Verification items for the finished model (mm, model axes). Coordinates: 2 decimals unless noted, no trailing zeros. Loops run counter-clockwise (first coordinate to the right, second up) from the corner with the lowest first, then second, coordinate; pieces in that order, holes last. Notation, with made-up numbers: (-16, 46.5) - (6, 46.5) arc R14 ccw to (6, 69.5) - close; hole circle Ø10 at (67.25, -30). An arc over 180 degrees is marked (long way). Answer as CSV lines item,"result". Start each with the question number.
1. Release check for a two-part mould opening along X. For faces 1 (the cylindrical face through (190.527, 25.813, 1.565)), 2 (the flat face through (166, 37, 3.175)) record: pulls with the +X half, pulls with the -X half, needs draft (parallel to the pull), parting line crosses it, or undercut.
2. Material ranges on line 1 (X direction, y = 12.5, z = 1.75); line 2 (X direction, y = 15.5, z = 0.4); line 3 (X direction, y = 22.5, z = 2.55), recorded low to high. Write a range as [from, to].
3. Cross-section at A-A (x = 323.85). Enter the section's corners in (y, z) (3 decimals), plus the area to 3 significant figures.
4. Cross-section at B-B (z = 2.6). State how many separate pieces and enclosed holes the cut face has, plus the area to 3 significant figures.
Autodesk Inventor part; units mm, degrees
ref_plane "YZ Plane" through (0, 0, 0) normal (1, 0, 0) x (0, 1, 0)
ref_plane "XZ Plane" through (0, 0, 0) normal (0, 1, 0) x (-1, 0, 0)
ref_plane "XY Plane" through (0, 0, 0) normal (0, 0, 1) x (1, 0, 0)
sketch "Sketch1" plane through (0, 0, 0) normal (0, 0, 1) x (1, 0, 0)
  line L0 (355.6, 50.8) -> (-19.05, 50.8)
  line L1 (12.7, 50.8) -> (12.7, 0) construction
  line L2 (0, 38.1) -> (12.7, 38.1) construction
  line L3 (0, 12.7) -> (12.7, 12.7) construction
  circle A0 centre (12.7, 38.1) radius 3.175
  circle A1 centre (12.7, 12.7) radius 3.175
  line L4 (168.275, 50.8) -> (168.275, 0) construction
  line L5 (-19.05, 50.8) -> (-19.05, 0)
  line L6 (355.6, 50.8) -> (355.6, 0)
  circle A2 centre (-9.525, 25.4) radius 3.175
  circle A3 centre (323.85, 38.1) radius 3.175
  circle A4 centre (323.85, 12.7) radius 3.175
  line L7 (355.6, 50.8) -> (355.6, 0)
  circle A5 centre (346.075, 25.4) radius 3.175
  line L8 (-19.05, 0) -> (355.6, 0)
  dimension "d0" = 374.65
  dimension "d3" = 12.7
  dimension "d4" = 25.4
  dimension "d5" = 6.35
  dimension "d6" = 6.35
  dimension "d10" = 6.35
  dimension "d11" = 31.75
extrude "Extrusion2" add sketch "Sketch1" along normal blind 3.175
sketch "Sketch3" plane through (0, 0, 3.175) normal (0, 0, 1) x (1, 0, 0)
  line L0 (-19.05, 50.8) -> (-19.05, 0)
  line L1 (-19.05, 25.4) -> (168.275, 25.4)
  line L2 (355.6, 50.8) -> (-19.05, 50.8)
  line L3 (168.275, 25.4) -> (168.275, 50.8)
  point P0 (0, 0)
hole "Hole1" at (168.275, 25.4, 3.175) direction (0, 0, -1) diameter 22.86 depth 25.4 tip angle 118
sketch "Sketch4" plane through (0, 0, 3.175) normal (0, 0, 1) x (1, 0, 0)
  circle A0 centre (168.275, 25.4) radius 11.43
  line L0 (168.275, 25.4) -> (142.875, 25.4)
  circle A1 centre (142.875, 25.4) radius 3.175
  line L1 (355.6, 50.8) -> (-19.05, 50.8)
  line L2 (168.275, 50.8) -> (168.275, 0)
  circle A2 centre (193.675, 25.4) radius 3.175
  point P0 (0, 0)
  dimension "d21" = 25.4
  dimension "d22" = 6.35
hole "Hole2" at (193.675, 25.4, 3.175) at (142.875, 25.4, 3.175) direction (0, 0, -1) diameter 6.35 depth 25.4 tip angle 118
sketch "Sketch5" plane through (0, 0, 3.175) normal (0, 0, 1) x (1, 0, 0)
  line L0 (355.6, 50.8) -> (-19.05, 50.8)
  line L1 (74.6506, 50.8) -> (74.6506, 0)
  line L2 (-19.05, 50.8) -> (-19.05, 0)
  line L3 (74.6506, 50.8) -> (74.6506, 44.45)
  line L4 (74.6506, 44.45) -> (74.6506, 25.4)
  circle A0 centre (74.6506, 44.45) radius 2.0701
  line L5 (74.6506, 25.4) -> (74.6506, 6.35)
  circle A1 centre (74.6506, 25.4) radius 2.0701
  circle A2 centre (74.6506, 6.35) radius 2.0701
  line L6 (168.275, 50.8) -> (168.275, 0)
  circle A3 centre (261.8994, 44.45) radius 2.0701
  circle A4 centre (261.8994, 25.4) radius 2.0701
  circle A5 centre (261.8994, 6.35) radius 2.0701
  point P0 (0, 0)
  dimension "d30" = 93.7006
  dimension "d31" = 6.35
  dimension "d32" = 19.05
  dimension "d33" = 4.1402
  dimension "d34" = 19.05
  dimension "d35" = 4.1402
  dimension "d36" = 4.1402
hole "Hole3" at (74.6506, 44.45, 3.175) at (74.6506, 25.4, 3.175) at (74.6506, 6.35, 3.175) at (261.8994, 44.45, 3.175) at (261.8994, 25.4, 3.175) at (261.8994, 6.35, 3.175) direction (0, 0, -1) diameter 4.1402 depth 25.4 tip angle 118
properties part number "slider-crossbeam" material "Aluminum 6061"
Values follow:
1,face 1,"undercut"
1,face 2,"needs draft"
2,line 1,"x = [-19.05, 9.53], [15.87, 320.68], [327.02, 355.6]"
2,line 2,"x = [-19.05, 11.2], [14.2, 162.56], [173.99, 322.35], [325.35, 355.6]"
2,line 3,"x = [-19.05, -10.82], [-8.23, 141.58], [144.17, 157.22], [179.33, 192.38], [194.97, 344.78], [347.37, 355.6]"
3,outline,"(0, 0) - (9.525, 0) - (9.525, 3.175) - (0, 3.175) - close; (15.875, 0) - (34.925, 0) - (34.925, 3.175) - (15.875, 3.175) - close; (41.275, 0) - (50.8, 0) - (50.8, 3.175) - (41.275, 3.175) - close"
3,area,"121 mm²"
4,separate pieces,"1"
4,enclosed holes,"15"
4,area,"18,300 mm²"
